Study the drawing (mm; zero at the part's minimum x, y, z) and answer. A direction names the side the tool comes from. Coordinates: 2 decimals unless noted, no trailing zeros. Order: outer loops, then holes, each group sorted by start corner. A loop starts at its lowest first (then second) coordinate and runs counter-clockwise, first axis right, second up. Notation, with made-up numbers: M -12.5,-11.75 L -8.5,-11.75 A23 ccw -8.5,13.25 Z; hole C 3.25,-36.75 d9. An arc over 180 degrees is marked long. One line per item, written item: value. Start each with the question number.
Q1. Straight lines are drawn through the part: line 1 along Y through (x, z) = (10.5, 5.5); line 2 along Z through (x, y) = (16.5, 7.75); line 3 along Y through (x, z) = (12, 1). For each, find the intervals that lie inside material, in ascending order. Write a range as [from, to].
Q2. This flat-tipped pin is pushed along its axis until it touches: pin 1 Ø2 at (x, y) = (13, 3.5) entering from -Z. Where does it stop, or does it pass through?
Q3. The part is cut by section C-C on x = 14.5. Give the vertices of the cut face in (y, z).
Q4. Determine the mould class of the marked faces 1, 2 and 3 for opening direction X: pulls with the +X half, pulls with the -X half, needs draft (parallel to the pull), parting line crosses it, or undercut.
Q5. The part is cut by section A-A on x = 10.5. Give the vertices of the cut face in (y, z), then the cut area to 3 significant figures.
Q6. The part is cut by section B-B on y = 8.25. Give the vertices of the cut face in (x, z).
Q7. For the marked faces 4 and 5, determine the directions among +Z, -Z, +X, -X, +Y, -Y from which every point of the face is accessible in a straight line to the end or side of a thin tool.
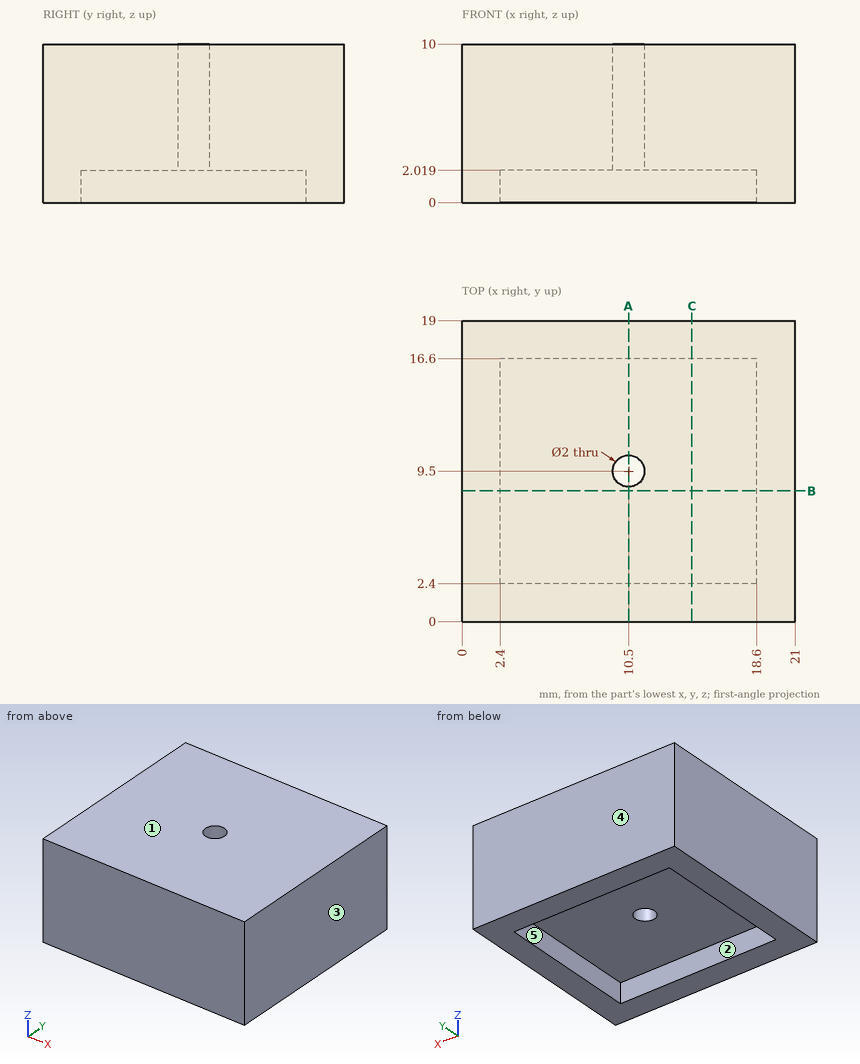
Output:
1. line 1: y = [0, 8.5], [10.5, 19]
1. line 2: z = [2.02, 10]
1. line 3: y = [0, 2.4], [16.6, 19]
2. pin 1: stops at z = 2.02
3. outline: M 0,0 L 2.4,0 L 2.4,2.02 L 16.6,2.02 L 16.6,0 L 19,0 L 19,10 L 0,10 Z
4. face 1: needs draft
4. face 2: undercut
4. face 3: pulls with the +X half
5. outline: M 0,0 L 2.4,0 L 2.4,2.02 L 8.5,2.02 L 8.5,10 L 0,10 Z; M 10.5,2.02 L 16.6,2.02 L 16.6,0 L 19,0 L 19,10 L 10.5,10 Z
5. area: 145 mm^2
6. outline: M 0,0 L 2.4,0 L 2.4,2.02 L 18.6,2.02 L 18.6,0 L 21,0 L 21,10 L 0,10 Z
7. face 4: +Z, -Z, +X, -X, +Y
7. face 5: -Z
